For this review, take the finished solid that the model builds, in its own axes (mm). Coordinates: 2 decimals unless noted, no trailing zeros. Loops run counter-clockwise (first coordinate to the right, second up) from the corner with the lowest first, then second, coordinate; pieces in that order, holes last. Notation, with made-up numbers: M 15.5,-32.5 L 69.5,-32.5 A23 cw 69.5,-4.5 Z; hole C 60.5,-29 d8. An arc over 180 degrees is marked long. Answer as a JSON object with one key per item and string values. Group by question number.
Item 1: Add section D-D (x = 146.5). State the section outline as (y, z) points.
Item 2: Add section B-B (z = 0.65). State the section outline as (x, y) points, then the cut area to 3 significant figures.
Item 3: Insertion check: pin 1 (14 mm diameter, centred on x = 25, y = 50, fed in from +Z). The pin has a flat end and moves straight along its axis. Give the tip position at first contact, or say it passes through.
Item 4: Add section A-A (x = 175). State the section outline as (y, z) points.
Item 5: Mouldability with a two-part tool opening along Y and no side actions: class faces 1 (the face through (170.64, 50.19, 1.97)), 2 (the face through (200, 30, 2)), 3 (the face through (2.85, 3.01, 1.97)) as +Y half, -Y half, draft (parallel to the pull), parting line (faces both ways), or undercut.
Item 6: Add section C-C (y = 67). State the section outline as (x, z) points, then the cut area to 3 significant figures.
Item 7: Wall thickness on L1, parallel to Y at x = 175, z = 1.25; L2, parallel to X at y = 63.5, z = 3.85; L3, parallel to Y at x = 138.5, z = 1.5: over which ranges is each line inside the solid? List them lowest first. Write a range as from..to.
from build123d import *

# Parameters (mm, degrees)
SKETCH1_R           = 4.365625
BOSS_EXTRUDE1_DEPTH = 4


with BuildPart() as part:
    # Sketch1 → Boss-Extrude1 (new body)
    with BuildSketch(Plane.XY):
        with BuildLine():
            Line((10, 0), (190, 0))
            ThreePointArc((190, 0), (197.071067812, 2.928932188), (200, 10))
            Line((200, 10), (200, 50))
            ThreePointArc((200, 50), (186.180339887, 72.360679775), (160, 70))
            ThreePointArc((160, 70), (100, 50), (40, 70))
            ThreePointArc((40, 70), (13.819660113, 72.360679775), (0, 50))
            Line((0, 50), (0, 10))
            ThreePointArc((0, 10), (2.928932188, 2.928932188), (10, 0))
        make_face()
        with Locations((25, 50)):
            Circle(SKETCH1_R, mode=Mode.SUBTRACT)
        with Locations((175, 50)):
            Circle(SKETCH1_R, mode=Mode.SUBTRACT)
    extrude(amount=BOSS_EXTRUDE1_DEPTH)


solid = part.part
From the geometry:
{
 "1": {"outline": "M 0,0 L 61.47,0 L 61.47,4 L 0,4 Z"},
 "2": {"outline": "M 0,10 A10 ccw 10,0 L 190,0 A10 ccw 200,10 L 200,50 A25 ccw 160,70 A100 cw 40,70 A25 ccw 0,50 Z; hole C 25,50 d8.73; hole C 175,50 d8.73", "area": "12,300 mm²"},
 "3": {"pin 1": "stops at z = 4"},
 "4": {"outline": "M 0,0 L 45.63,0 L 45.63,4 L 0,4 Z; M 54.37,0 L 75,0 L 75,4 L 54.37,4 Z"},
 "5": {"face 1": "undercut", "face 2": "draft", "face 3": "-Y half"},
 "6": {"outline": "M 6.67,0 L 44.22,0 L 44.22,4 L 6.67,4 Z; M 155.78,0 L 193.33,0 L 193.33,4 L 155.78,4 Z", "area": "300 mm²"},
 "7": {"L1": "y = 0..45.63, 54.37..75", "L2": "x = 3.96..49.82, 150.18..196.04", "L3": "y = 0..57.71"}
}
